Could you check a few things on this model? Use its own coordinates, in mm. Give positions to 0.01 mm unless a question says otherwise; leave off trailing zeros. Loops run counter-clockwise (first coordinate to the right, second up) from the corner with the lowest first, then second, coordinate; pieces in that order, holes last.
1. Thinking about a two-plate mould opening in X: for faces 1 (the cylindrical face through (0.358, 2.465, -47.727)), 2 (the flat face through (-42.704, 2.465, -36.822)), 3 (the cylindrical face through (0.085, 2.465, -64.467)), which applies, +X half, -X half, draft (parallel to the pull), parting line (faces both ways), or undercut?
2. I need wall thicknesses on line 1 along Z through (x, y) = (0, 3.25); line 2 along X through (y, z) = (2.05, -2); line 3 along X through (y, z) = (3.8, -45). Which ranges of each line are inside material? Lowest first, please.
3. Imagine slicing it at D-D (z = -45). List the corners of the cut face in (x, y) for me.
4. Imagine slicing it at B-B (z = -20). List the corners of the cut face in (x, y) for me.
5. Imagine slicing it at A-A (x = 0). List the corners of the cut face in (y, z) for me.
6. For P1, Ø4.5, axis at x = -77.93, z = -1.59, coming from the -Y side, with a flat end and sliding along its axis, tell me the tip position at first contact or that it passes through.
7. Imagine slicing it at C-C (y = 2.55). List the corners of the cut face in (x, z) for me.
```python
from build123d import *

# Parameters (mm, degrees)
BOSS_EXTRUDE1_DEPTH  = 5
M5_CLEARANCE_HOLE1_D = 5.5
M5_CLEARANCE_HOLE2_D = 5.5


with BuildPart() as part:
    # Sketch2 → Boss-Extrude1 (new body)
    with BuildSketch(Plane(origin=(0, 0, 0), x_dir=(1, 0, 0), z_dir=(0, 1, 0))):
        with BuildLine():
            Line((-5.72861373, 62.663882494), (-80.72861373, 10.24579688))
            ThreePointArc((-80.72861373, 10.24579688), (-84.538480676, -0.953622176), (-75, -7.950725842))
            Line((-75, -7.950725842), (75, -7.950725842))
            ThreePointArc((75, -7.950725842), (84.538480676, -0.953622176), (80.72861373, 10.24579688))
            Line((80.72861373, 10.24579688), (5.72861373, 62.663882494))
            ThreePointArc((5.72861373, 62.663882494), (0, 64.467359772), (-5.72861373, 62.663882494))
        make_face()
    extrude(amount=BOSS_EXTRUDE1_DEPTH)

    # M5 Clearance Hole1 (through all)
    with Locations(Plane(origin=(0, 5, 0), x_dir=(1, 0, 0), z_dir=(0, 1, 0))):
        with Locations((0, 45), (0, 20)):
            Hole(M5_CLEARANCE_HOLE1_D / 2)

    # M5 Clearance Hole2 (through all)
    with Locations(Plane(origin=(0, 5, 0), x_dir=(1, 0, 0), z_dir=(0, 1, 0))):
        with Locations((-77.928915997, 1.587505431)):
            m5_clearance_hole2 = Hole(M5_CLEARANCE_HOLE2_D / 2)

    # Mirror1: M5 Clearance Hole2 across plane
    add(m5_clearance_hole2.mirror(Plane(origin=(0, 0, 0), x_dir=(0, 0, 1), z_dir=(1, 0, 0))), mode=Mode.SUBTRACT)


solid = part.part
```
Derived:
1. face 1: undercut
1. face 2: -X half
1. face 3: parting line
2. line 1: z = -64.47 to -47.75, -42.25 to -22.75, -17.25 to 7.95
2. line 2: x = -85 to -80.65, -75.21 to 75.21, 80.65 to 85
2. line 3: x = -31 to -2.75, 2.75 to 31
3. outline: (-31, 0) - (-2.75, 0) - (-2.75, 5) - (-31, 5) - close; (2.75, 0) - (31, 0) - (31, 5) - (2.75, 5) - close
4. outline: (-66.77, 0) - (-2.75, 0) - (-2.75, 5) - (-66.77, 5) - close; (2.75, 0) - (66.77, 0) - (66.77, 5) - (2.75, 5) - close
5. outline: (0, -64.47) - (5, -64.47) - (5, -47.75) - (0, -47.75) - close; (0, -42.25) - (5, -42.25) - (5, -22.75) - (0, -22.75) - close; (0, -17.25) - (5, -17.25) - (5, 7.95) - (0, 7.95) - close
6. P1: passes through
7. outline: (-80.73, -10.25) - (-5.73, -62.66) arc R10 ccw to (5.73, -62.66) - (80.73, -10.25) arc R10 ccw to (75, 7.95) - (-75, 7.95) arc R10 ccw to start; hole circle Ø5.5 at (-77.93, -1.59); hole circle Ø5.5 at (0, -45); hole circle Ø5.5 at (0, -20); hole circle Ø5.5 at (77.93, -1.59)
